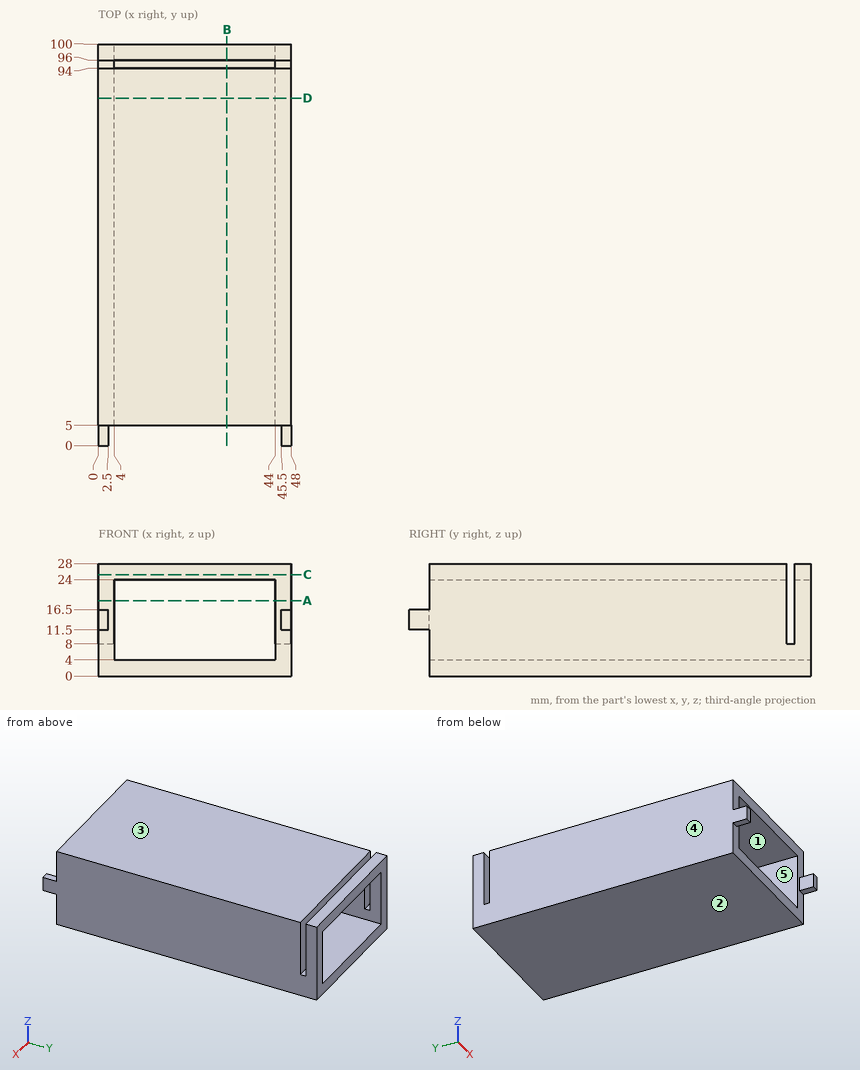
Job drawing, mm, ordinate dimensions from the low corner. One solid piece. A direction names the side the tool comes from. Coordinates: 2 decimals unless noted, no trailing zeros. Order: outer loops, then holes, each group sorted by start corner. A loop starts at its lowest first (then second) coordinate and runs counter-clockwise, first axis right, second up. Notation, with made-up numbers: (33, 4) -> (58, 4) arc R18 cw to (58, 39) -> close; hole circle Ø1 at (-5.5, -17). An arc over 180 degrees is marked (long way). Return JSON: item names as keys, results as strings. Group by question number.
Item 1: Saw through at C-C on z = 25.25. Write the cut outline in (x, y), then the cut area to 3 significant figures.
Item 2: Flat gauge pins, fed straight in: P1, Ø0.6, axis at x = 2, y = 95.5, coming from the +Z side; P2, Ø14, axis at x = 14.5, z = 9, coming from the -Y side; P3, Ø2, axis at x = 1, y = 1.5, coming from the -Z side. Where does each tip first touch, or does it go through?
Item 3: Saw through at A-A on z = 18.75. Write the cut outline in (x, y), then the cut area to 3 significant figures.
Item 4: Saw through at B-B on x = 32. Write the cut outline in (y, z), then the cut area to 3 significant figures.
Item 5: Wall check: line 1 along X through (y, z) = (11, 21.75); line 2 along Z through (x, y) = (31, 7); line 3 along Y through (x, z) = (2, 13.25). Give the ranges that are in metal, low to high. Write a range as [from, to].
Item 6: Tool access for the marked faces 1 and 2: list every direction of +Z, -Z, +X, -X, +Y, -Y with a clear straight run to the whole face (end or side of a thin tool).
Item 7: Pull direction Z, two halves, no side cores. Call the marked faces 3, 4 and 5: pulls with the +Z half, pulls with the -Z half, needs draft (parallel to the pull), parting line crosses it, or undercut.
Item 8: Saw through at D-D on y = 86.5. Write the cut outline in (x, z).
Values found:
{
 "1": {"outline": "(0, 5) -> (48, 5) -> (48, 94) -> (0, 94) -> close; (0, 96) -> (48, 96) -> (48, 100) -> (0, 100) -> close", "area": "4,460 mm2"},
 "2": {"P1": "stops at z = 8", "P2": "stops at y = 5", "P3": "stops at z = 11.5"},
 "3": {"outline": "(0, 5) -> (4, 5) -> (4, 94) -> (0, 94) -> close; (0, 96) -> (4, 96) -> (4, 100) -> (0, 100) -> close; (44, 5) -> (48, 5) -> (48, 94) -> (44, 94) -> close; (44, 96) -> (48, 96) -> (48, 100) -> (44, 100) -> close", "area": "744 mm2"},
 "4": {"outline": "(5, 0) -> (100, 0) -> (100, 4) -> (5, 4) -> close; (5, 24) -> (94, 24) -> (94, 28) -> (5, 28) -> close; (96, 24) -> (100, 24) -> (100, 28) -> (96, 28) -> close", "area": "752 mm2"},
 "5": {"line 1": "x = [0, 4], [44, 48]", "line 2": "z = [0, 4], [24, 28]", "line 3": "y = [0, 94], [96, 100]"},
 "6": {"face 1": "+Y, -Y", "face 2": "-Z, +X, -X, +Y, -Y"},
 "7": {"face 3": "pulls with the +Z half", "face 4": "needs draft", "face 5": "undercut"},
 "8": {"outline": "(0, 0) -> (48, 0) -> (48, 28) -> (0, 28) -> close; hole (4, 4) -> (44, 4) -> (44, 24) -> (4, 24) -> close"}
}
